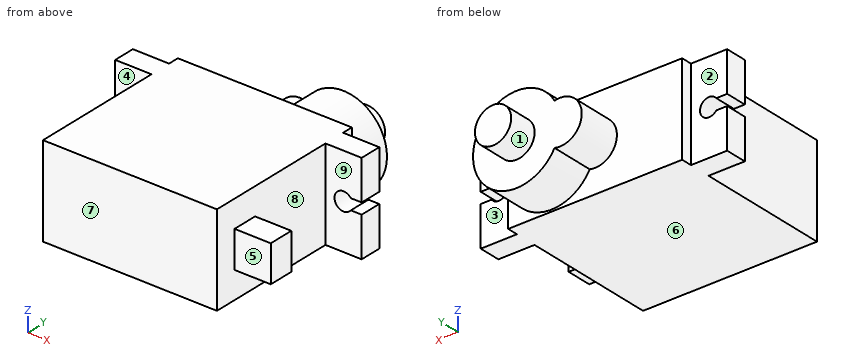
Autodesk Inventor part; units mm, degrees
ref_plane "YZ Plane" through (0, 0, 0) normal (1, 0, 0) x (0, 1, 0)
ref_plane "XZ Plane" through (0, 0, 0) normal (0, 1, 0) x (-1, 0, 0)
ref_plane "XY Plane" through (0, 0, 0) normal (0, 0, 1) x (1, 0, 0)
sketch "Sketch1" plane through (0, 0, 0) normal (0, 0, 1) x (1, 0, 0)
  line L0 (-2.5, 0) -> (2.5, 0)
  line L1 (2.5, 0) -> (2.5, -4)
  line L2 (2.5, -4) -> (-2.5, -4)
  line L3 (-2.5, -4) -> (-2.5, 0)
  line L4 (6, -4) -> (-9, -4)
  line L5 (-9, -4) -> (-9, -10)
  line L6 (-9, -10) -> (6, -10)
  line L7 (6, -10) -> (6, -4)
  line L8 (6, -10) -> (-18, -10)
  line L9 (-18, -10) -> (-18, -33)
  line L10 (-18, -33) -> (6, -33)
  line L11 (6, -33) -> (6, -10)
  line L12 (-18, -11.5) -> (-23, -11.5)
  line L13 (-23, -11.5) -> (-23, -14.5)
  line L14 (-23, -14.5) -> (-18, -14.5)
  line L15 (-18, -14.5) -> (-18, -11.5)
  line L16 (6, -11.5) -> (11, -11.5)
  line L17 (11, -11.5) -> (11, -14.5)
  line L18 (11, -14.5) -> (6, -14.5)
  line L19 (6, -14.5) -> (6, -11.5)
  line L20 (-6, -33) -> (-6, -10) construction
  point P0 (0, 0)
  point P1 (0, -4)
  point P2 (11, -13)
  point P3 (-23, -13)
  point P4 (-9, -7)
  point P5 (0, 0)
  point P6 (-18, -14.5)
  point P7 (6, -14.5)
  dimension "d0" = 5
  dimension "d1" = 4
  dimension "d2" = 6
  dimension "d3" = 6
  dimension "d4" = 24
  dimension "d6" = 34
  dimension "d7" = 9
  dimension "d8" = 1.5
  dimension "d9" = 3
  dimension "d31" = 18.5
extrude "Extrusion1" add sketch "Sketch1" along normal mid plane 12.5 contours L6 L11 L10 L9 L8 | L16 L17 L18 L11 | L9 L14 L13 L12
sketch "Sketch2" plane through (-18, -10, 6.25) normal (0, 1, 0) x (1, 0, 0)
  circle A0 centre (18, 6.25) radius 6
  line L0 (24, 12.5) -> (24, 0) construction
  circle A1 centre (12, 6.25) radius 3
  line L1 (0, 12.5) -> (0, 0) construction
  point P0 (9, 6.25)
  point P1 (0, 6.25)
  point P2 (12.75, 9.1547)
  point P3 (12.75, 3.3453)
  dimension "d12" = 9
extrude "Extrusion2" add sketch "Sketch2" along normal blind 6
sketch "Sketch3" plane through (-18, -4, 6.25) normal (0, 1, 0) x (1, 0, 0)
  circle A0 centre (18, 6.25) radius 2.5
  dimension "d15" = 5
extrude "Extrusion3" add sketch "Sketch3" along normal blind 4
sketch "Sketch4" plane through (6, -33, 6.25) normal (1, 0, 0) x (0, 0, -1)
  line L0 (3.7222, 6.5) -> (8.7778, 6.5)
  line L1 (8.7778, 6.5) -> (8.7778, 3)
  line L2 (8.7778, 3) -> (3.7222, 3)
  line L3 (3.7222, 3) -> (3.7222, 6.5)
  line L4 (0, 0) -> (0, 18.5) construction
  line L5 (0, 6.5) -> (3.7222, 6.5) construction
  line L6 (8.7778, 6.5) -> (12.5, 6.5) construction
  line L7 (12.5, 18.5) -> (12.5, 0) construction
  line L8 (12.5, 0) -> (0, 0) construction
  line L9 (12.5, 18.5) -> (0, 18.5) construction
  point P0 (6.25, 33)
  point P1 (6.25, 18.5)
  point P2 (6.25, 6.5)
  dimension "d18" = 3
  dimension "d19" = 12
extrude "Extrusion4" add sketch "Sketch4" along normal blind 5
sketch "Sketch5" plane through (6, -11.5, 6.25) normal (0, 1, 0) x (1, 0, 0)
  line L0 (-29, 12.5) -> (-29, 0) construction
  line L1 (-24, 0) -> (-29, 0) construction
  line L2 (-24, 12.5) -> (-24, 0) construction
  line L3 (-29, 12.5) -> (-24, 12.5) construction
  line L4 (0, 12.5) -> (0, 0) construction
  line L5 (5, 0) -> (0, 0) construction
  line L6 (5, 12.5) -> (5, 0) construction
  line L7 (0, 12.5) -> (5, 12.5) construction
  line L8 (-29, 6.25) -> (5, 6.25) construction
  line L9 (5, 3.7222) -> (5, 8.7778) construction
  circle A0 centre (-26.5, 6.25) radius 1.25
  circle A1 centre (2.5, 6.25) radius 1.25
  line L10 (-12, 6.25) -> (-12, 12.5) construction
  line L11 (-27.5, 5.5) -> (-29, 5.5)
  line L12 (-29, 5.5) -> (-29, 7)
  line L13 (-29, 7) -> (-27.5, 7)
  line L14 (-27.5, 7) -> (-27.5, 5.5)
  line L15 (3.5, 7) -> (5, 7)
  line L16 (5, 7) -> (5, 5.5)
  line L17 (5, 5.5) -> (3.5, 5.5)
  line L18 (3.5, 5.5) -> (3.5, 7)
  line L19 (3.5, 7) -> (5, 5.5) construction
  line L20 (5, 7) -> (3.5, 5.5) construction
  point P0 (-6, 6.25)
  point P1 (4.25, 6.25)
  point P2 (3.5, 5.5)
  dimension "d22" = 2.5
  dimension "d23" = 29
  dimension "d24" = 1.5
  dimension "d25" = 1.5
extrude "Extrusion5" cut sketch "Sketch5" against normal blind 3
sketch "草圖7" plane through (0, 0, 0) normal (0, 1, 0) x (1, 0, 0)
  line L0 (-23, 0.75) -> (-21.5, 0.75)
  arc A0 (-21.5, -0.75) -> (-21.5, 0.75) centre (-20.5, 0) ccw
  line L1 (-21.5, -0.75) -> (-23, -0.75)
  line L2 (-23, -0.75) -> (-23, -6.25)
  line L3 (-18, -6.25) -> (-23, -6.25)
  line L4 (-18, 6.25) -> (-18, -6.25)
  line L5 (-23, 6.25) -> (-18, 6.25)
  line L6 (-23, 6.25) -> (-23, 0.75)
  line L7 (-18, 6.25) -> (-18, -6.25)
  line L8 (6, -6.25) -> (-18, -6.25)
  line L9 (6, 0) -> (6, -6.25)
  arc A1 (-5.25, -2.9047) -> (6, 0) centre (0, 0) ccw
  arc A2 (-5.25, 2.9047) -> (-5.25, -2.9047) centre (-6, 0) ccw
  arc A3 (6, 0) -> (-5.25, 2.9047) centre (0, 0) ccw
  line L10 (6, 6.25) -> (6, 0)
  line L11 (-18, 6.25) -> (6, 6.25)
  circle A4 centre (0, 0) radius 2.5
  arc A5 (-5.25, -2.9047) -> (-5.25, 2.9047) centre (0, 0) ccw
  arc A6 (-5.25, 2.9047) -> (-5.25, -2.9047) centre (-6, 0) ccw
  circle A7 centre (0, 0) radius 2.5
  line L12 (11, -0.75) -> (9.5, -0.75)
  arc A8 (9.5, 0.75) -> (9.5, -0.75) centre (8.5, 0) ccw
  line L13 (9.5, 0.75) -> (11, 0.75)
  line L14 (11, 6.25) -> (11, 0.75)
  line L15 (6, 6.25) -> (11, 6.25)
  line L16 (6, 6.25) -> (6, -6.25)
  line L17 (11, -6.25) -> (6, -6.25)
  line L18 (11, -0.75) -> (11, -6.25)
  point P0 (0, 0)
sketch "Sketch6" plane through (0, 0, 0) normal (0, 1, 0) x (1, 0, 0)
  circle A0 centre (0, 0) radius 2.5
  circle A1 centre (0, 0) radius 10
  point P0 (0, 0)
  dimension "d28" = 20
properties part number "S"
Build history of the part. All positions in model axes, mm. Face numbers are marked on the shaded views. A direction names the side the tool comes from. Round coordinates to 2 decimals unless told otherwise and drop trailing zeros. Write each loop counter-clockwise with the first axis right and the second up, starting at its lowest first coordinate (ties: lowest second). Pieces come first, ordered by that corner, then holes. Notation, with made-up numbers: (40, 48) -> (98, 48) arc R29 cw to (98, 69) -> close; hole circle Ø8 at (-5, 6.25). An arc over 180 degrees is marked (long way). Use one line per item in the form item = value.
Q1. Band-saw the part on A-A, the plane x = -20.5. Write the cut outline in (y, z).
Conclusion:
outline = (-14.5, -6.25) -> (-11.5, -6.25) -> (-11.5, -1.25) -> (-14.5, -1.25) -> close; (-14.5, 1.25) -> (-11.5, 1.25) -> (-11.5, 6.25) -> (-14.5, 6.25) -> close
Q2. Two-plate mould, pull along Y, no slides. Class the marked faces 6, 7, 8 and 9: released by +Y, released by -Y, zero draft, split by the parting line, or undercut.
Conclusion:
face_6 = zero draft
face_7 = released by -Y
face_8 = undercut
face_9 = undercut
Q3. Drill centre lines: L1, parallel to Z at x = -20.5, y = -12.55; L2, parallel to X at y = -13.45, z = 0; L3, parallel to X at y = -30, z = 3.25. Where is each one in solid material? Low to high.
Conclusion:
L1 = -6.25 to -1.25, 1.25 to 6.25
L2 = -19.25 to 7.25
L3 = -18 to 6
Q4. Drop flat-ended pins along their axis: P1, Ø5.5, axis at x = 8.5, z = -3, coming from the +Y side; P2, Ø2.5, axis at x = 7.5, z = -2.5, coming from the -Y side; P3, Ø1.5, axis at x = -20.5, z = 2.5, coming from the -Y side. Give the stop position or say it passes through.
Conclusion:
P1 = -10
P2 = -30
P3 = -14.5
Q5. Band-saw the part on C-C, the plane x = 8.5. Write the cut outline in (y, z).
Conclusion:
outline = (-30, -2.53) -> (-26.5, -2.53) -> (-26.5, 2.53) -> (-30, 2.53) -> close; (-14.5, -6.25) -> (-11.5, -6.25) -> (-11.5, -1.25) -> (-14.5, -1.25) -> close; (-14.5, 1.25) -> (-11.5, 1.25) -> (-11.5, 6.25) -> (-14.5, 6.25) -> close
Q6. Tool access for the marked faces 1, 2, 3, 4 and 5: list every direction of +Z, -Z, +X, -X, +Y, -Y with a clear straight run to the whole face (end or side of a thin tool).
Conclusion:
face_1 = +Y
face_2 = +Z, -Z, -X, +Y
face_3 = +Z, -Z, +X, +Y
face_4 = +Z, -Z, -X, -Y
face_5 = +Z, -Z, +X, -Y
Q7. Band-saw the part on B-B, the plane y = -27.5. Write the cut outline in (x, z), then the cut area to 3 significant figures.
Conclusion:
outline = (-18, -6.25) -> (6, -6.25) -> (6, -2.53) -> (11, -2.53) -> (11, 2.53) -> (6, 2.53) -> (6, 6.25) -> (-18, 6.25) -> close
area = 325 mm²
Q8. Band-saw the part on D-D, the plane z = 3.5. Write the cut outline in (x, y), then the cut area to 3 significant figures.
Conclusion:
outline = (-23, -14.5) -> (-18, -14.5) -> (-18, -33) -> (6, -33) -> (6, -14.5) -> (11, -14.5) -> (11, -11.5) -> (6, -11.5) -> (6, -10) -> (4.87, -10) -> (4.87, -4) -> (-4.87, -4) -> (-4.87, -10) -> (-18, -10) -> (-18, -11.5) -> (-23, -11.5) -> close
area = 640 mm²
